from build123d import *

# Parameters (mm, degrees)
F0_W     = 254
F0_H     = 203.2
F1_DEPTH = 3.175
F2_R     = 25.4
F3_R     = 9.525
F3_R_2   = 6.746875
F4_DEPTH = 3.176


with BuildPart() as f1:
    # F0 (on Top) → F1 (new body)
    with BuildSketch(Plane.XY):
        Rectangle(F0_W, F0_H)
    extrude(amount=F1_DEPTH)

    # F2
    f2_edges = [f1.edges().sort_by_distance(p)[0] for p in [
        (127, 101.6, 1.5875),
        (-127, 101.6, 1.5875),
        (127, -101.6, 1.5875),
        (-127, -101.6, 1.5875),
    ]]
    fillet(f2_edges, radius=F2_R)

    # F3 (on face) → F4 (cut, through all)
    with BuildSketch(Plane.XY.offset(3.175)):
        with Locations((0, 76.2)):
            Circle(F3_R)
        with Locations((0, -76.2)):
            Circle(F3_R)
        with Locations((-101.6, 76.2)):
            Circle(F3_R_2)
        with Locations((-101.6, -76.2)):
            Circle(F3_R_2)
        with Locations((101.6, 76.2)):
            Circle(F3_R_2)
        with Locations((101.6, -76.2)):
            Circle(F3_R_2)
    extrude(amount=-F4_DEPTH, mode=Mode.SUBTRACT)


solid = f1.part
The model under review builds one solid part; all positions refer to its coordinate system, in mm. Give positions to 0.01 mm unless a question says otherwise; leave off trailing zeros. Order: outer loops, then holes, each group sorted by start corner. A loop starts at its lowest first (then second) coordinate and runs counter-clockwise, first axis right, second up. Notation, with made-up numbers: (42.5, 32.5) -> (79.5, 32.5) arc R21 cw to (79.5, 61.5) -> close; hole circle Ø9 at (29, -35). An arc over 180 degrees is marked (long way). Write item = value, one per line. Start each with the question number.
(1) For L1, parallel to Y at x = 0, z = 1.7 (3 decimals); L2, parallel to Y at x = 8.5, z = 1.7; L3, parallel to X at y = 71, z = 2.1, list the stretches that pass through material, from the lowest coordinate up. Write a range as from..to.
(2) Draft analysis for pull direction Y (two halves, no side actions). For faces 1 (the cylindrical face through (108.035, 78.227, 1.61)), 2 (the flat face through (-2, 1, 0)), 3 (the cylindrical face through (4.4, 67.75, 1.61)), 4 (the cylindrical face through (-119.76, -93.96, 1.61)), state which applies: +Y half, -Y half, draft (parallel to the pull), parting line (faces both ways), or undercut.
(3) Take a section at C-C (y = -73.5). Write out the cut boundary in (x, z) (3 decimals), plus the area to 3 significant figures.
(4) Take a section at D-D (x = -105.5). Write out the cut boundary in (y, z) (3 decimals), plus the area to 3 significant figures.
(5) For pin 1 Ø8 at (x, y) = (-101.6, 76.2) entering from -Z; pin 2 Ø21.5 at (x, y) = (101.6, -76.2) entering from -Z, all flat-tipped, find the tip position at first contact; note any pin that passes through.
(6) Take a section at A-A (x = 0). Write out the cut boundary in (y, z) (3 decimals).
(7) Take a section at B-B (z = 1.45). Write out the cut boundary in (x, y) (3 decimals).
Returned:
q1.L1 = -101.6..-85.725, -66.675..66.675, 85.725..101.6
q1.L2 = -101.6..-80.5, -71.9..71.9, 80.5..101.6
q1.L3 = -127..-105.9, -97.3..-7.98, 7.98..97.3, 105.9..127
q2.face_1 = undercut
q2.face_2 = draft
q2.face_3 = undercut
q2.face_4 = -Y half
q3.outline = (-127, 0) -> (-107.783, 0) -> (-107.783, 3.175) -> (-127, 3.175) -> close; (-95.417, 0) -> (-9.134, 0) -> (-9.134, 3.175) -> (-95.417, 3.175) -> close; (9.134, 0) -> (95.417, 0) -> (95.417, 3.175) -> (9.134, 3.175) -> close; (107.783, 0) -> (127, 0) -> (127, 3.175) -> (107.783, 3.175) -> close
q3.area = 670 mm²
q4.outline = (-101.299, 0) -> (-81.705, 0) -> (-81.705, 3.175) -> (-101.299, 3.175) -> close; (-70.695, 0) -> (70.695, 0) -> (70.695, 3.175) -> (-70.695, 3.175) -> close; (81.705, 0) -> (101.299, 0) -> (101.299, 3.175) -> (81.705, 3.175) -> close
q4.area = 573 mm²
q5.pin_1 = through
q5.pin_2 = 0
q6.outline = (-101.6, 0) -> (-85.725, 0) -> (-85.725, 3.175) -> (-101.6, 3.175) -> close; (-66.675, 0) -> (66.675, 0) -> (66.675, 3.175) -> (-66.675, 3.175) -> close; (85.725, 0) -> (101.6, 0) -> (101.6, 3.175) -> (85.725, 3.175) -> close
q7.outline = (-127, -76.2) arc R25.4 ccw to (-101.6, -101.6) -> (101.6, -101.6) arc R25.4 ccw to (127, -76.2) -> (127, 76.2) arc R25.4 ccw to (101.6, 101.6) -> (-101.6, 101.6) arc R25.4 ccw to (-127, 76.2) -> close; hole circle Ø13.494 at (-101.6, -76.2); hole circle Ø13.494 at (-101.6, 76.2); hole circle Ø19.05 at (0, -76.2); hole circle Ø19.05 at (0, 76.2); hole circle Ø13.494 at (101.6, -76.2); hole circle Ø13.494 at (101.6, 76.2)
